Verification items for the finished model (mm, model axes). A direction names the side the tool comes from. Coordinates: 2 decimals unless noted, no trailing zeros. Write each loop counter-clockwise with the first axis right and the second up, starting at its lowest first coordinate (ties: lowest second). Pieces come first, ordered by that corner, then holes. Notation, with made-up numbers: (-35, 52.25) -> (-24, 52.25) arc R25 ccw to (-24, 70.25) -> close; hole circle Ø3 at (81.5, 33.25). An arc over 180 degrees is marked (long way). Use CSV: the item, a comma, the result in double quotes.
Autodesk Inventor part; units mm, degrees
ref_plane "YZ Plane" through (0, 0, 0) normal (1, 0, 0) x (0, 1, 0)
ref_plane "XZ Plane" through (0, 0, 0) normal (0, 1, 0) x (-1, 0, 0)
ref_plane "XY Plane" through (0, 0, 0) normal (0, 0, 1) x (1, 0, 0)
sketch "Sketch1" plane through (0, 0, 0) normal (0, 0, 1) x (1, 0, 0)
  line L0 (0, 0) -> (164.5, 0)
  line L1 (164.5, 0) -> (164.5, 9)
  line L2 (164.5, 9) -> (0, 9)
  line L3 (0, 9) -> (0, 0)
  circle A0 centre (99, 4) radius 1.6
  circle A1 centre (159.5, 4) radius 1.6
  circle A2 centre (147, 4) radius 1.6
  circle A3 centre (15, 4) radius 1.6
  circle A4 centre (7, 4) radius 1.6
  dimension "d1" = 9
  dimension "d2" = 90
  dimension "d6" = 3.2
  dimension "d7" = 3.2
  dimension "d9" = 60.5
  dimension "d26" = 3.2
  dimension "d27" = 48
  dimension "d28" = 3.2
  dimension "d32" = 15
  dimension "d33" = 5
  dimension "d61" = 3.2
  dimension "d62" = 8
  dimension "d63" = 12.5
  dimension "d108" = 4
  dimension "d109" = 4
  dimension "d111" = 4
  dimension "d112" = 4
  dimension "d113" = 4
ref_plane "Work Plane2" through (0, 0, 0) normal (0, -1, 0) x (1, 0, 0)
sketch "Sketch2" plane through (0, 0, 0) normal (0, -1, 0) x (1, 0, 0)
  circle A0 centre (52, 8) radius 1.6
  circle A1 centre (125, 8) radius 1.6
  circle A2 centre (88.5, 8) radius 1.6
  point P0 (0, 0)
  point P1 (52, 0)
  dimension "d13" = 3.2
  dimension "d15" = 3.2
  dimension "d17" = 3.2
  dimension "d18" = 36.5
  dimension "d64" = 52
  dimension "d65" = 36.5
  dimension "d114" = 8
  dimension "d115" = 73
ref_plane "Work Plane1" through (0, 0, 11) normal (0, 0, 1) x (1, 0, 0)
extrude "klocek" add sketch "Sketch1" along normal blind 11
ref_plane "Work Plane3" through (0, 0, 0) normal (0, -1, 0) x (1, 0, 0)
extrude "prowadzenie osi" cut sketch "Sketch2" against normal up to next
ref_plane "Work Plane4" through (0, 0, 0) normal (0, -1, 0) x (1, 0, 0)
sketch "Sketch7" plane through (0, 0, 0) normal (0, -1, 0) x (1, 0, 0)
  line L0 (0, 11) -> (0, 1)
  line L1 (0, 11) -> (164.5, 11)
  line L2 (0, 11) -> (40, 11)
  line L3 (40, 11) -> (0, 1)
  point P0 (0, -1.8333)
  dimension "d86" = 10
  dimension "d87" = 40
sketch "Sketch8" plane through (0, 0, 0) normal (0, -1, 0) x (1, 0, 0)
  line L0 (164.5, 0) -> (164.5, 11)
  line L1 (164.5, 11) -> (164.5, 1)
  line L2 (164.5, 11) -> (0, 11)
  line L3 (164.5, 11) -> (134.5, 11)
  line L4 (134.5, 11) -> (164.5, 1)
  point P0 (0, 0)
  point P1 (40.8333, 11)
  dimension "d80" = 10
  dimension "d81" = 30
extrude "przedni skos" cut sketch "Sketch7" against normal up to next
extrude "tylni skos" cut sketch "Sketch8" against normal up to next
ref_plane "Work Plane7" through (0, 0, 11) normal (0, 0, 1) x (1, 0, 0)
sketch "Sketch5" plane through (0, 0, 11) normal (0, 0, 1) x (1, 0, 0)
  circle A0 centre (99, 4) radius 1.6
  line L0 (95.5936, 4) -> (97.2968, 6.95)
  line L1 (97.2968, 6.95) -> (100.7032, 6.95)
  line L2 (100.7032, 6.95) -> (102.4064, 4)
  line L3 (102.4064, 4) -> (100.7032, 1.05)
  line L4 (100.7032, 1.05) -> (97.2968, 1.05)
  line L5 (97.2968, 1.05) -> (95.5936, 4)
  point P0 (119.5, 5)
  dimension "d98" = 5.9
extrude "hex insert middle" cut sketch "Sketch5" against normal blind 3
ref_plane "Work Plane6" through (0, 0, 11) normal (0, 0, 1) x (1, 0, 0)
sketch "Sketch9" plane through (0, 0, 11) normal (0, 0, 1) x (1, 0, 0)
  circle A0 centre (147, 4) radius 1.6
  line L0 (150.4064, 4) -> (148.7032, 1.05)
  line L1 (148.7032, 1.05) -> (145.2968, 1.05)
  line L2 (145.2968, 1.05) -> (143.5936, 4)
  line L3 (143.5936, 4) -> (145.2968, 6.95)
  line L4 (145.2968, 6.95) -> (148.7032, 6.95)
  line L5 (148.7032, 6.95) -> (150.4064, 4)
  point P0 (0, 0)
  point P1 (153, 5)
  dimension "d99" = 5.9
extrude "hex insert rear 1" cut sketch "Sketch9" against normal blind 7.5
ref_plane "Work Plane5" through (0, 0, 11) normal (0, 0, 1) x (1, 0, 0)
sketch "Sketch10" plane through (0, 0, 11) normal (0, 0, 1) x (1, 0, 0)
  circle A0 centre (159.5, 4) radius 1.6
  line L0 (162.45, 5.7032) -> (162.45, 2.2968)
  line L1 (162.45, 2.2968) -> (159.5, 0.5936)
  line L2 (159.5, 0.5936) -> (156.55, 2.2968)
  line L3 (156.55, 2.2968) -> (156.55, 5.7032)
  line L4 (156.55, 5.7032) -> (159.5, 7.4064)
  line L5 (159.5, 7.4064) -> (162.45, 5.7032)
  line L6 (164.5, 0) -> (134.5, 0)
  point P0 (0, 0)
  dimension "d118" = 5.9
extrude "hex insert rear 2" cut sketch "Sketch10" against normal up to next contours A0 | L0 L1 L2 L3 L4 L5
sketch "Sketch13" plane through (0, 0, 11) normal (0, 0, 1) x (1, 0, 0)
  circle A0 centre (7, 4) radius 1.6
  line L0 (10.4064, 4) -> (8.7032, 1.05)
  line L1 (8.7032, 1.05) -> (5.2968, 1.05)
  line L2 (5.2968, 1.05) -> (3.5936, 4)
  line L3 (3.5936, 4) -> (5.2968, 6.95)
  line L4 (5.2968, 6.95) -> (8.7032, 6.95)
  line L5 (8.7032, 6.95) -> (10.4064, 4)
  dimension "d123" = 5.9
extrude "hex insert front 1" cut sketch "Sketch13" against normal through all
sketch "Sketch16" plane through (0, 0, 11) normal (0, 0, 1) x (1, 0, 0)
  circle A0 centre (15, 4) radius 1.6
  line L0 (18.4064, 4) -> (16.7032, 1.05)
  line L1 (16.7032, 1.05) -> (13.2968, 1.05)
  line L2 (13.2968, 1.05) -> (11.5936, 4)
  line L3 (11.5936, 4) -> (13.2968, 6.95)
  line L4 (13.2968, 6.95) -> (16.7032, 6.95)
  line L5 (16.7032, 6.95) -> (18.4064, 4)
  point P0 (0, 0)
  dimension "d93" = 5.9
extrude "hex insert front 2" cut sketch "Sketch16" against normal blind 9
sketch "Sketch17" plane through (0, 0, 0) normal (0, 0, -1) x (-1, 0, 0)
  line L0 (-164.5, 9) -> (0, 9)
  line L1 (0, 0) -> (-2, 0)
  line L2 (-2, 0) -> (-2, 9)
  line L3 (-2, 9) -> (0, 9)
  line L4 (0, 9) -> (0, 0)
  dimension "d122" = 2
extrude "ciecie przod" cut sketch "Sketch17" against normal up to next
sketch "Sketch18" plane through (40, 0, 11) normal (0, -1, 0) x (1, 0, 0)
  line L0 (9.5, 0) -> (9.5, -2)
  line L1 (9.5, -2) -> (-7.5, -2)
  line L2 (-7.5, -2) -> (-7.5, 0)
  line L3 (-7.5, 0) -> (9.5, 0)
  line L4 (94.5, 0) -> (0, 0)
  circle A0 centre (12, -3) radius 1.6
  line L5 (-40, -11) -> (124.5, -11)
  point P0 (-35, -11)
  dimension "d102" = 2
  dimension "d103" = 17
  dimension "d104" = 2.5
extrude "sensor linii" cut sketch "Sketch18" against normal blind 7.3 contours L0 L1 L2 L3
properties part number "wheel_support_v5_left_narrow_with_line_sensor"
1) Set-up check for faces 4 (the flat face through (82, 0, 4)), 5 (the flat face through (161, 1.46, 1.06)), 6 (the flat face through (99, 6.95, 10)): record each of +Z, -Z, +X, -X, +Y, -Y from which the full face is reachable in a straight line by a thin tool's end or side.
Return value:
face 4,"+Z, -Z, +X, -X, -Y"
face 5,"+Z, -Z"
face 6,"+Z"
2) Mould release check, pull along Z, two halves, no side actions. Record for faces 1 (the flat face through (148.5, 5.4, 3.5)), 2 (the cylindrical face through (53.48, 4.44, 7.39)), 3 (the flat face through (158.05, 1.43, 1.44)): released by +Z, released by -Z, zero draft, split by the parting line, or undercut.
Return value:
face 1,"released by +Z"
face 2,"undercut"
face 3,"zero draft"
3) Cross-section at B-B (x = 52). Record the boundary of the cut face in (y, z), plus the area to 3 significant figures.
Return value:
outline,"(0, 0) -> (9, 0) -> (9, 6.4) -> (0, 6.4) -> close; (0, 9.6) -> (9, 9.6) -> (9, 11) -> (0, 11) -> close"
area,"70.2 mm2"
4) Cross-section at C-C (x = 99). Record the boundary of the cut face in (y, z), plus the area to 3 significant figures.
Return value:
outline,"(0, 0) -> (2.4, 0) -> (2.4, 8) -> (1.05, 8) -> (1.05, 11) -> (0, 11) -> close; (5.6, 0) -> (9, 0) -> (9, 11) -> (6.95, 11) -> (6.95, 8) -> (5.6, 8) -> close"
area,"55.7 mm2"
5) Scan lines: L1, parallel to Z at x = 88.5, y = 5.25; L2, parallel to Z at x = 35.5, y = 2.75; L3, parallel to Y at x = 147, z = 2.7. Record each from-to range of solid material in increasing order.
Return value:
L1,"0 to 6.4, 9.6 to 11"
L2,"0 to 9"
L3,"0 to 2.4, 5.6 to 9"
6) Cross-section at A-A (x = 15). Record the boundary of the cut face in (y, z), plus the area to 3 significant figures.
Return value:
outline,"(0, 0) -> (2.4, 0) -> (2.4, 2) -> (1.05, 2) -> (1.05, 4.75) -> (0, 4.75) -> close; (5.6, 0) -> (9, 0) -> (9, 4.75) -> (6.95, 4.75) -> (6.95, 2) -> (5.6, 2) -> close"
area,"20.1 mm2"
7) Gauge pin test, flat ends, axial feed: pin 1 (1.6 mm diameter, centred on x = 7.5, z = 2, fed in from -Y); pin 2 (0.6 mm diameter, centred on y = 4.5, z = 10.5, fed in from -X); pin 3 (4 mm diameter, centred on x = 99, y = 4, fed in from +Z); pin 4 (4.5 mm diameter, centred on x = 16.5, y = 3, fed in from +Z). Record the tip position at first contact, or that the pin passes through.
Return value:
pin 1,"y = 0"
pin 2,"x = 49.5"
pin 3,"z = 8"
pin 4,"z = 5.69"
